```python
from build123d import *

# Parameters (mm, degrees)
Y_KSEKLIK_EKSTR_ZYON1_DEPTH = 2
IZIM2_R                     = 2
KES_EKSTR_ZYON1_DEPTH       = 2


with BuildPart() as part:
    # Çizim1 → Yükseklik-Ekstrüzyon1 (new body)
    with BuildSketch(Plane.YZ):
        with BuildLine():
            Line((78.698599078, 126.350175115), (53.698599078, 126.350175115))
            ThreePointArc((53.698599078, 126.350175115), (52.991492297, 126.643068334), (52.698599078, 127.350175115))
            Line((52.698599078, 127.350175115), (52.698599078, 129.350175115))
            ThreePointArc((52.698599078, 129.350175115), (49.698599078, 132.350175115), (46.698599078, 129.350175115))
            Line((46.698599078, 129.350175115), (46.698599078, 127.350175115))
            ThreePointArc((46.698599078, 127.350175115), (46.40570586, 126.643068334), (45.698599078, 126.350175115))
            Line((45.698599078, 126.350175115), (-43.301400922, 126.350175115))
            ThreePointArc((-43.301400922, 126.350175115), (-44.008507703, 126.643068334), (-44.301400922, 127.350175115))
            Line((-44.301400922, 127.350175115), (-44.301400922, 129.350175115))
            ThreePointArc((-44.301400922, 129.350175115), (-47.301400922, 132.350175115), (-50.301400922, 129.350175115))
            Line((-50.301400922, 129.350175115), (-50.301400922, 127.350175115))
            ThreePointArc((-50.301400922, 127.350175115), (-50.59429414, 126.643068334), (-51.301400922, 126.350175115))
            Line((-51.301400922, 126.350175115), (-76.301400922, 126.350175115))
            ThreePointArc((-76.301400922, 126.350175115), (-79.129828046, 125.17860224), (-80.301400922, 122.350175115))
            Line((-80.301400922, 122.350175115), (-80.301400922, 90.350175115))
            ThreePointArc((-80.301400922, 90.350175115), (-80.59429414, 89.643068334), (-81.301400922, 89.350175115))
            Line((-81.301400922, 89.350175115), (-85.301400922, 89.350175115))
            ThreePointArc((-85.301400922, 89.350175115), (-88.301400922, 86.350175115), (-85.301400922, 83.350175115))
            Line((-85.301400922, 83.350175115), (-81.301400922, 83.350175115))
            ThreePointArc((-81.301400922, 83.350175115), (-80.59429414, 83.057281896), (-80.301400922, 82.350175115))
            Line((-80.301400922, 82.350175115), (-80.301400922, -82.649824885))
            ThreePointArc((-80.301400922, -82.649824885), (-80.59429414, -83.356931666), (-81.301400922, -83.649824885))
            Line((-81.301400922, -83.649824885), (-85.301400922, -83.649824885))
            ThreePointArc((-85.301400922, -83.649824885), (-88.301400922, -86.649824885), (-85.301400922, -89.649824885))
            Line((-85.301400922, -89.649824885), (-81.301400922, -89.649824885))
            ThreePointArc((-81.301400922, -89.649824885), (-80.59429414, -89.942718104), (-80.301400922, -90.649824885))
            Line((-80.301400922, -90.649824885), (-80.301400922, -122.649824885))
            ThreePointArc((-80.301400922, -122.649824885), (-79.129828046, -125.47825201), (-76.301400922, -126.649824885))
            Line((-76.301400922, -126.649824885), (-51.301400922, -126.649824885))
            ThreePointArc((-51.301400922, -126.649824885), (-50.59429414, -126.942718104), (-50.301400922, -127.649824885))
            Line((-50.301400922, -127.649824885), (-50.301400922, -129.649824885))
            ThreePointArc((-50.301400922, -129.649824885), (-47.301400922, -132.649824885), (-44.301400922, -129.649824885))
            Line((-44.301400922, -129.649824885), (-44.301400922, -127.649824885))
            ThreePointArc((-44.301400922, -127.649824885), (-44.008507703, -126.942718104), (-43.301400922, -126.649824885))
            Line((-43.301400922, -126.649824885), (45.698599078, -126.649824885))
            ThreePointArc((45.698599078, -126.649824885), (46.40570586, -126.942718104), (46.698599078, -127.649824885))
            Line((46.698599078, -127.649824885), (46.698599078, -129.649824885))
            ThreePointArc((46.698599078, -129.649824885), (49.698599078, -132.649824885), (52.698599078, -129.649824885))
            Line((52.698599078, -129.649824885), (52.698599078, -127.649824885))
            ThreePointArc((52.698599078, -127.649824885), (52.991492297, -126.942718104), (53.698599078, -126.649824885))
            Line((53.698599078, -126.649824885), (78.698599078, -126.649824885))
            ThreePointArc((78.698599078, -126.649824885), (81.527026203, -125.47825201), (82.698599078, -122.649824885))
            Line((82.698599078, -122.649824885), (82.698599078, -90.649824885))
            ThreePointArc((82.698599078, -90.649824885), (82.991492297, -89.942718104), (83.698599078, -89.649824885))
            Line((83.698599078, -89.649824885), (87.698599078, -89.649824885))
            ThreePointArc((87.698599078, -89.649824885), (90.698599078, -86.649824885), (87.698599078, -83.649824885))
            Line((87.698599078, -83.649824885), (83.698599078, -83.649824885))
            ThreePointArc((83.698599078, -83.649824885), (82.991492297, -83.356931666), (82.698599078, -82.649824885))
            Line((82.698599078, -82.649824885), (82.698599078, 82.350175115))
            ThreePointArc((82.698599078, 82.350175115), (82.991492297, 83.057281896), (83.698599078, 83.350175115))
            Line((83.698599078, 83.350175115), (87.698599078, 83.350175115))
            ThreePointArc((87.698599078, 83.350175115), (90.698599078, 86.350175115), (87.698599078, 89.350175115))
            Line((87.698599078, 89.350175115), (83.698599078, 89.350175115))
            ThreePointArc((83.698599078, 89.350175115), (82.991492297, 89.643068334), (82.698599078, 90.350175115))
            Line((82.698599078, 90.350175115), (82.698599078, 122.350175115))
            ThreePointArc((82.698599078, 122.350175115), (81.527026203, 125.17860224), (78.698599078, 126.350175115))
        make_face()
    extrude(amount=Y_KSEKLIK_EKSTR_ZYON1_DEPTH)

    # Çizim2 → Kes-Ekstrüzyon1 (cut)
    with BuildSketch(Plane.YZ.offset(2)):
        with Locations(Location((-47.301400922, 129.350175115, 0), (0, 0, 270))):
            Circle(IZIM2_R)
    kes_ekstr_zyon1 = extrude(amount=-KES_EKSTR_ZYON1_DEPTH, mode=Mode.SUBTRACT)

    # Çizim-Çoğaltma1: Kes-Ekstrüzyon1 at 7 more places
    with Locations((0, 97, 0), (0, 135, -43), (0, -38, -43), (0, -38, -216), (0, 0, -259), (0, 97, -259), (0, 135, -216)):
        add(kes_ekstr_zyon1, mode=Mode.SUBTRACT)


solid = part.part
```
Check sheet for the modelled part. Datum: model origin and axes. Units: mm. Round coordinates to 2 decimals unless told otherwise and drop trailing zeros. Write each loop counter-clockwise with the first axis right and the second up, starting at its lowest first coordinate (ties: lowest second). Pieces come first, ordered by that corner, then holes. Notation, with made-up numbers: M 78.25,83.5 L 104.25,83.5 A22 ccw 104.25,105.5 Z; hole C 50,32.25 d11. An arc over 180 degrees is marked long. Write item = value, one per line. Start each with the question number.
1. Gauge pin test, flat ends, axial feed: pin 1 (3 mm diameter, centred on y = -47.3, z = -129.65, fed in from -X); pin 2 (1 mm diameter, centred on x = 1, y = 64, fed in from -Z); pin 3 (0.6 mm diameter, centred on x = 0.5, y = -84, fed in from -Z); pin 4 (0.6 mm diameter, centred on x = 1.5, z = 100, fed in from -Y). Record the tip position at first contact, or that the pin passes through.
2. Section check C-C, the plane z = -37.5. Record the cut outline in (x, y), then the cut area to 3 significant figures.
3. Section check B-B, the plane x = 0.75. State how many separate pieces and enclosed holes the cut face has, then the cut area to 3 significant figures.
4. Section check A-A, the plane y = -39. Record the cut outline in (x, z).
5. Scan lines: line 1 (Z direction, x = 0.25, y = 12); line 2 (Y direction, x = 0.55, z = -39.5); line 3 (Z direction, x = 1.1, y = 46). Record each from-to range of solid material in increasing order. Write a range as [from, to].
Results found:
q1.pin_1 = through
q1.pin_2 = -126.65
q1.pin_3 = -89.65
q1.pin_4 = -80.3
q2.outline = M 0,-80.3 L 2,-80.3 L 2,82.7 L 0,82.7 Z
q2.area = 326 mm^2
q3.separate_pieces = 1
q3.enclosed_holes = 8
q3.area = 41,400 mm^2
q4.outline = M 0,-126.65 L 2,-126.65 L 2,126.35 L 0,126.35 Z
q5.line_1 = [-126.65, 126.35]
q5.line_2 = [-80.3, 82.7]
q5.line_3 = [-126.7, 126.4]
